Work out the finished part from the listing and answer in its coordinate system (mm). Round coordinates to 2 decimals unless told otherwise and drop trailing zeros. Loops run counter-clockwise (first coordinate to the right, second up) from the corner with the lowest first, then second, coordinate; pieces in that order, holes last. Notation, with made-up numbers: (16.25, -32.75) - (59.25, -32.75) arc R19 cw to (59.25, 3.25) - close; hole circle Ø1 at (54.5, -35). An arc over 180 degrees is marked (long way). Return JSON: item names as keys, results as strings.
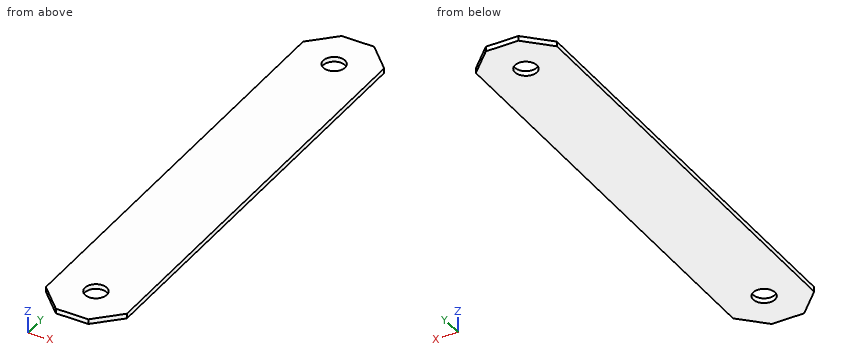
Autodesk Fusion 360 part; units mm, degrees
sketch "Sketch1" plane through (0, 0, 0) normal (0, 0, 1) x (1, 0, 0)
  line L0 (-10, 60) -> (10, 60)
  line L1 (10, 60) -> (10, -60)
  line L2 (10, -60) -> (-10, -60)
  line L3 (-10, -60) -> (-10, 60)
  line L4 (-10, 60) -> (10, -60) construction
  line L5 (10, 60) -> (-10, -60) construction
  circle A0 centre (0, -50) radius 2.7
  line L6 (0, -50) -> (-10, -50) construction
  line L7 (0, -50) -> (0, -60) construction
  line L8 (90, 0) -> (-64.2965, 0) construction
  circle A1 centre (0, 50) radius 2.7
  dimension "d1" = 120
  dimension "d2" = 20
  dimension "d3" = 5.4
extrude "Extrude1" add sketch "Sketch1" along normal blind 1.2
chamfer "Chamfer1" distance 6 angle 45 2 edges at (10, -60, 0.6) (-10, -60, 0.6)
chamfer "Chamfer1" distance 6 angle 45 2 edges at (10, 60, 0.6) (-10, 60, 0.6)
1) Section D-D (x = -8.25) is taken. Give the vertices of the cut face in (y, z), and give its area (3 significant figures).
Verdict:
{"outline": "(-55.75, 0) - (55.75, 0) - (55.75, 1.2) - (-55.75, 1.2) - close", "area": "134 mm2"}
2) Section B-B (y = 50) is taken. Give the vertices of the cut face in (x, z), and give its area (3 significant figures).
Verdict:
{"outline": "(-10, 0) - (-2.7, 0) - (-2.7, 1.2) - (-10, 1.2) - close; (2.7, 0) - (10, 0) - (10, 1.2) - (2.7, 1.2) - close", "area": "17.5 mm2"}
3) Section A-A (x = 0) is taken. Give the vertices of the cut face in (y, z).
Verdict:
{"outline": "(-60, 0) - (-52.7, 0) - (-52.7, 1.2) - (-60, 1.2) - close; (-47.3, 0) - (47.3, 0) - (47.3, 1.2) - (-47.3, 1.2) - close; (52.7, 0) - (60, 0) - (60, 1.2) - (52.7, 1.2) - close"}
4) Section C-C (z = 0.85) is taken. Give the vertices of the cut face in (x, y).
Verdict:
{"outline": "(-10, -54) - (-4, -60) - (4, -60) - (10, -54) - (10, 54) - (4, 60) - (-4, 60) - (-10, 54) - close; hole circle Ø5.4 at (0, -50); hole circle Ø5.4 at (0, 50)"}
5) Find the intervals of material crossed by L1, parallel to Y at x = 0, z = 0.95; L2, parallel to Y at x = -1.5, z = 0.2 (3 decimals); L3, parallel to X at y = 48.5, z = 0.75 (3 decimals), in increasing order.
Verdict:
{"L1": "y = -60 to -52.7, -47.3 to 47.3, 52.7 to 60", "L2": "y = -60 to -52.245, -47.755 to 47.755, 52.245 to 60", "L3": "x = -10 to -2.245, 2.245 to 10"}
